The model under review builds one solid part; all positions refer to its coordinate system, in mm. Face numbers are marked on the shaded views. A direction names the side the tool comes from. Give positions to 0.01 mm unless a question says otherwise; leave off trailing zeros. Loops run counter-clockwise (first coordinate to the right, second up) from the corner with the lowest first, then second, coordinate; pieces in that order, holes last. Notation, with made-up numbers: (-33, 64) -> (19, 64) arc R22 ccw to (19, 99) -> close; hole circle Ø9 at (7.5, 13.25). An arc over 180 degrees is marked (long way). Write each question's results on one line, items separated by ' | '. Start each with the question number.
Q1. We need section A-A (z = 13). Write out the cut boundary in (x, y), plus the area to 3 significant figures.
Q2. Machinability: for the marked faces 1, 2 and 3, which of the approach directions +Z, -Z, +X, -X, +Y, -Y give a long, thin tool a straight path to every point of the face, cutting with its end or side? Answer none if there is none.
Q3. We need section B-B (y = 24.5). Write out the cut boundary in (x, z).
Q4. We need section D-D (y = 56.5). Write out the cut boundary in (x, z), plus the area to 3 significant figures.
Q5. Insertion check: pin 1 Ø6 at (y, z) = (34.5, 13) entering from -X; pin 2 Ø15 at (x, y) = (19, 21) entering from -Z; pin 3 Ø2 at (x, y) = (5.5, 28) entering from +Z. Each pin has a flat end and moves straight along its axis. Give the tip position at first contact, or say it passes through.
Q6. We need section C-C (x = 6.4). Write out the cut boundary in (y, z), plus the area to 3 significant figures.
Q7. Wall thickness on L1, parallel to Y at x = 6.4, z = 3.6; L2, parallel to Y at x = 33, z = 13; L3, parallel to Z at x = 23.5, y = 58.5: over which ranges is each line inside the solid? List them lowest first. Write a range as [from, to].
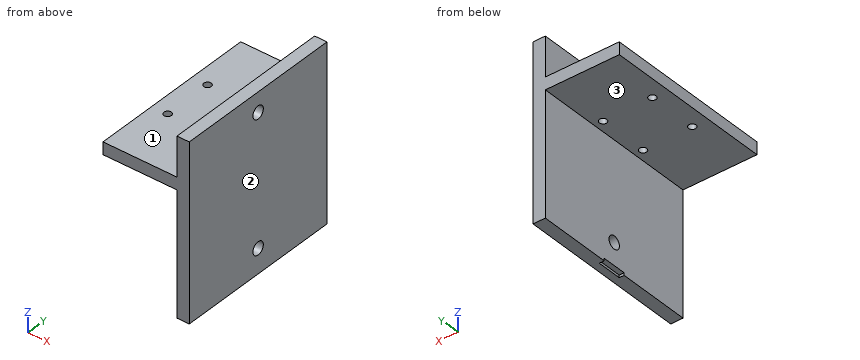
from build123d import *

# Parameters (mm, degrees)
EXTRUDE_1_DEPTH     = 69
HOLE_WIZARD_1_D     = 3
SKETCH_5_R          = 2.6
CUT_EXTRUDE_1_DEPTH = 10
SKETCH_6_R          = 2.6
CUT_EXTRUDE_2_DEPTH = 10
SKETCH_8_W          = 2
SKETCH_8_H          = 10
CUT_EXTRUDE_4_DEPTH = 2


with BuildPart() as part:
    # 草图1 → 凸台-拉伸1 (new body)
    with BuildSketch(Plane(origin=(0, 0, 0), x_dir=(1, 0, 0), z_dir=(0, 1, 0))):
        Polygon((30, 0), (30, 50), (35, 50), (35, -21), (30, -21), (30, -5), (0, -5), (0, 0), align=None)
    extrude(amount=EXTRUDE_1_DEPTH)

    # 孔1 (through all)
    with Locations(Plane.XY.offset(5)):
        with Locations((26.4, 44.5), (26.4, 24.5), (6.4, 44.5), (6.4, 24.5)):
            Hole(HOLE_WIZARD_1_D / 2)

    # 草图5 → 切除-拉伸1 (cut)
    with BuildSketch(Plane.ZY.offset(-30)):
        with Locations((13, 34.5)):
            Circle(SKETCH_5_R)
    extrude(amount=-CUT_EXTRUDE_1_DEPTH, mode=Mode.SUBTRACT)

    # 草图6 → 切除-拉伸2 (cut)
    with BuildSketch(Plane.ZY.offset(-30)):
        with Locations((-40, 34.5)):
            Circle(SKETCH_6_R)
    extrude(amount=-CUT_EXTRUDE_2_DEPTH, mode=Mode.SUBTRACT)

    # 草图8 → 切除-拉伸4 (cut)
    with BuildSketch(Plane.ZY.offset(-30)):
        with Locations((-50, 34.5)):
            Rectangle(SKETCH_8_W, SKETCH_8_H)
    extrude(amount=-CUT_EXTRUDE_4_DEPTH, mode=Mode.SUBTRACT)


solid = part.part
Output:
1) outline: (30, 0) -> (35, 0) -> (35, 31.9) -> (30, 31.9) -> close; (30, 37.1) -> (35, 37.1) -> (35, 69) -> (30, 69) -> close | area: 319 mm2
2) face 1: +Z, -X, +Y, -Y | face 2: +Z, -Z, +X, +Y, -Y | face 3: -Z, -X, +Y, -Y
3) outline: (0, 0) -> (4.9, 0) -> (4.9, 5) -> (0, 5) -> close; (7.9, 0) -> (24.9, 0) -> (24.9, 5) -> (7.9, 5) -> close; (27.9, 0) -> (30, 0) -> (30, -50) -> (35, -50) -> (35, 21) -> (30, 21) -> (30, 5) -> (27.9, 5) -> close
4) outline: (0, 0) -> (30, 0) -> (30, -50) -> (35, -50) -> (35, 21) -> (30, 21) -> (30, 5) -> (0, 5) -> close | area: 505 mm2
5) pin 1: x = 30 | pin 2: z = 0 | pin 3: z = 5
6) outline: (0, 0) -> (23, 0) -> (23, 5) -> (0, 5) -> close; (26, 0) -> (43, 0) -> (43, 5) -> (26, 5) -> close; (46, 0) -> (69, 0) -> (69, 5) -> (46, 5) -> close | area: 315 mm2
7) L1: [0, 23], [26, 43], [46, 69] | L2: [0, 31.9], [37.1, 69] | L3: [0, 5]
